Check sheet for the modelled part. Datum: model origin and axes. Units: mm. Give positions to 0.01 mm unless a question says otherwise; leave off trailing zeros. Order: outer loops, then holes, each group sorted by start corner. A loop starts at its lowest first (then second) coordinate and runs counter-clockwise, first axis right, second up. Notation, with made-up numbers: (64, 21) -> (101, 21) arc R25 ccw to (101, 35) -> close; hole circle Ø10 at (75.25, 10.5). An arc over 180 degrees is marked (long way). Write each question's results on one line, items separated by ' | '.
from build123d import *

# Parameters (mm, degrees)
PAD002_DEPTH      = 2
PAD002_DEPTH_BACK = 2
SKETCH_W          = 25
SKETCH_H          = 75
PAD_DEPTH         = 1


with BuildPart() as body002:
    # Sketch003 → Pad002 (new body, two sides)
    with BuildSketch(Plane.XY) as pad002_sk:
        Polygon((12.5, 46.875), (9.375, 28.125), (15.625, 28.125), align=None)
    extrude(amount=PAD002_DEPTH)
    extrude(pad002_sk.sketch, amount=-PAD002_DEPTH_BACK)


with BuildPart() as body:
    # Sketch → Pad (new body)
    with BuildSketch(Plane.XY):
        with Locations((12.5, 37.5)):
            Rectangle(SKETCH_W, SKETCH_H)
    extrude(amount=PAD_DEPTH)

    # Boolean: cut Body002
    add(body002.part, mode=Mode.SUBTRACT)


solid = body.part
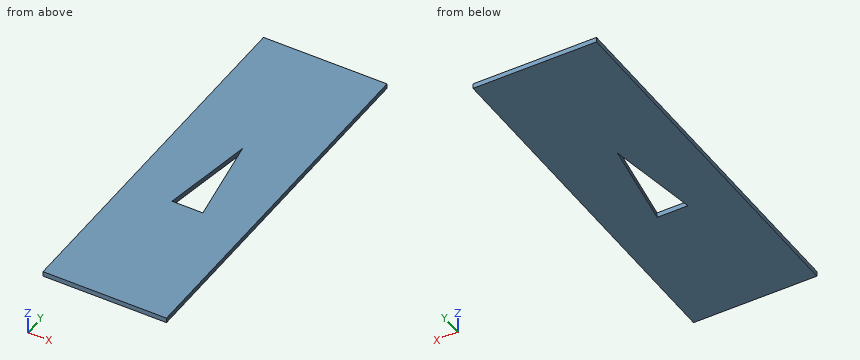
1. Section check B-B on y = 45. Record the cut outline in (x, z), then the cut area to 3 significant figures.
Verdict:
outline: (0, 0) -> (12.19, 0) -> (12.19, 1) -> (0, 1) -> close; (12.81, 0) -> (25, 0) -> (25, 1) -> (12.81, 1) -> close | area: 24.4 mm^2
2. Section check A-A on z = 0.85. Record the cut outline in (x, y) (3 decimals).
Verdict:
outline: (0, 0) -> (25, 0) -> (25, 75) -> (0, 75) -> close; hole (9.375, 28.125) -> (15.625, 28.125) -> (12.5, 46.875) -> close
3. Material ranges on probe 1 along X at (y, z) = (36, 0.7), recorded low to high. Write a range as from..to.
Verdict:
probe 1: x = 0..10.69, 14.31..25
4. Section check C-C on x = 14. Record the cut outline in (y, z) (3 decimals), then the cut area to 4 significant figures.
Verdict:
outline: (0, 0) -> (28.125, 0) -> (28.125, 1) -> (0, 1) -> close; (37.875, 0) -> (75, 0) -> (75, 1) -> (37.875, 1) -> close | area: 65.25 mm^2
